The model under review builds one solid part; all positions refer to its coordinate system, in mm. Round coordinates to 2 decimals unless told otherwise and drop trailing zeros. Loops run counter-clockwise (first coordinate to the right, second up) from the corner with the lowest first, then second, coordinate; pieces in that order, holes last. Notation, with made-up numbers: (31.25, 35.25) -> (86.25, 35.25) arc R20 cw to (86.25, 61.25) -> close; hole circle Ø11 at (16, 73.5). An arc over 180 degrees is marked (long way). Use CSV: the item, a comma, the result in double quotes. Start each with the question number.
```python
from build123d import *

# Parameters (mm, degrees)
SKETCH1_W           = 91
SKETCH1_H           = 97.3
BOSS_EXTRUDE1_DEPTH = 1.6
SKETCH2_W           = 11
SKETCH2_H           = 13
CUT_EXTRUDE1_DEPTH  = 1.6
SKETCH3_R           = 1.5
CUT_EXTRUDE2_DEPTH  = 1.6


with BuildPart() as part:
    # Sketch1 → Boss-Extrude1 (new body)
    with BuildSketch(Plane(origin=(0, 0, 0), x_dir=(1, 0, 0), z_dir=(0, 1, 0))):
        Rectangle(SKETCH1_W, SKETCH1_H)
    extrude(amount=BOSS_EXTRUDE1_DEPTH)

    # Sketch2 → Cut-Extrude1 (cut)
    with BuildSketch(Plane(origin=(0, 1.6, 0), x_dir=(1, 0, 0), z_dir=(0, 1, 0))):
        with Locations((-40, 42.15)):
            Rectangle(SKETCH2_W, SKETCH2_H)
        with Locations((40, 42.15)):
            Rectangle(SKETCH2_W, SKETCH2_H)
        with Locations((-40, -42.15)):
            Rectangle(SKETCH2_W, SKETCH2_H)
        with Locations((40, -42.15)):
            Rectangle(SKETCH2_W, SKETCH2_H)
    extrude(amount=-CUT_EXTRUDE1_DEPTH, mode=Mode.SUBTRACT)

    # Sketch3 → Cut-Extrude2 (cut)
    with BuildSketch(Plane(origin=(0, 1.6, 0), x_dir=(1, 0, 0), z_dir=(0, 1, 0))):
        with Locations((-30.5, 45.8)):
            Circle(SKETCH3_R)
        with Locations((30.5, 45.8)):
            Circle(SKETCH3_R)
    cut_extrude2 = extrude(amount=-CUT_EXTRUDE2_DEPTH, mode=Mode.SUBTRACT)

    # Mirror1: Cut-Extrude2 across plane
    add(cut_extrude2.mirror(Plane.XY), mode=Mode.SUBTRACT)


solid = part.part
```
1. Clearance check with flat-ended pins moving along their axes: P1, Ø0.8, axis at x = 38, y = 0.5, coming from the +Z side; P2, Ø2.5, axis at x = -30.5, z = 45.8, coming from the -Y side; P3, Ø0.5, axis at y = 1, z = 39.5, coming from the +X side; P4, Ø0.5, axis at x = -39, y = 0.5, coming from the -Z side. State where each tip first meets the part, or that it passes through.
2. For line 1 along X through (y, z) = (1, -45.8); line 2 along Z through (x, y) = (-30.5, 1.25); line 3 along Z through (x, y) = (-42, 0.1), list the stretches that pass through material, from the lowest coordinate up. Write a range as from..to.
3. Take a section at D-D, the plane z = -38.5. Give the boundary of the cut face in (x, y), then the cut area to 3 significant figures.
4. Take a section at C-C, the plane y = 0.3. Give the boundary of the cut face in (x, z), then the cut area to 3 significant figures.
5. Take a section at A-A, the plane x = -30.5. Give the boundary of the cut face in (y, z).
6. The part is to be moulded in two halves that separate along X. For faces 1 (the face through (29, 0.81, -45.87)), 2 (the face through (-1, 0, -1)), 3 (the face through (29, 0.81, 45.87)), say which applies: pulls with the +X half, pulls with the -X half, needs draft (parallel to the pull), parting line crosses it, or undercut.
7. Take a section at B-B, the plane z = 45.8. Give the boundary of the cut face in (x, y).
Results:
1,P1,"z = 35.65"
1,P2,"through"
1,P3,"x = 34.5"
1,P4,"z = -35.65"
2,line 1,"-34.5..-32, -29..29, 32..34.5"
2,line 2,"-48.65..-47.3, -44.3..44.3, 47.3..48.65"
2,line 3,"-35.65..35.65"
3,outline,"(-34.5, 0) -> (34.5, 0) -> (34.5, 1.6) -> (-34.5, 1.6) -> close"
3,area,"110 mm²"
4,outline,"(-45.5, -35.65) -> (-34.5, -35.65) -> (-34.5, -48.65) -> (34.5, -48.65) -> (34.5, -35.65) -> (45.5, -35.65) -> (45.5, 35.65) -> (34.5, 35.65) -> (34.5, 48.65) -> (-34.5, 48.65) -> (-34.5, 35.65) -> (-45.5, 35.65) -> close; hole circle Ø3 at (-30.5, -45.8); hole circle Ø3 at (-30.5, 45.8); hole circle Ø3 at (30.5, -45.8); hole circle Ø3 at (30.5, 45.8)"
4,area,"8,250 mm²"
5,outline,"(0, -48.65) -> (1.6, -48.65) -> (1.6, -47.3) -> (0, -47.3) -> close; (0, -44.3) -> (1.6, -44.3) -> (1.6, 44.3) -> (0, 44.3) -> close; (0, 47.3) -> (1.6, 47.3) -> (1.6, 48.65) -> (0, 48.65) -> close"
6,face 1,"undercut"
6,face 2,"needs draft"
6,face 3,"undercut"
7,outline,"(-34.5, 0) -> (-32, 0) -> (-32, 1.6) -> (-34.5, 1.6) -> close; (-29, 0) -> (29, 0) -> (29, 1.6) -> (-29, 1.6) -> close; (32, 0) -> (34.5, 0) -> (34.5, 1.6) -> (32, 1.6) -> close"
